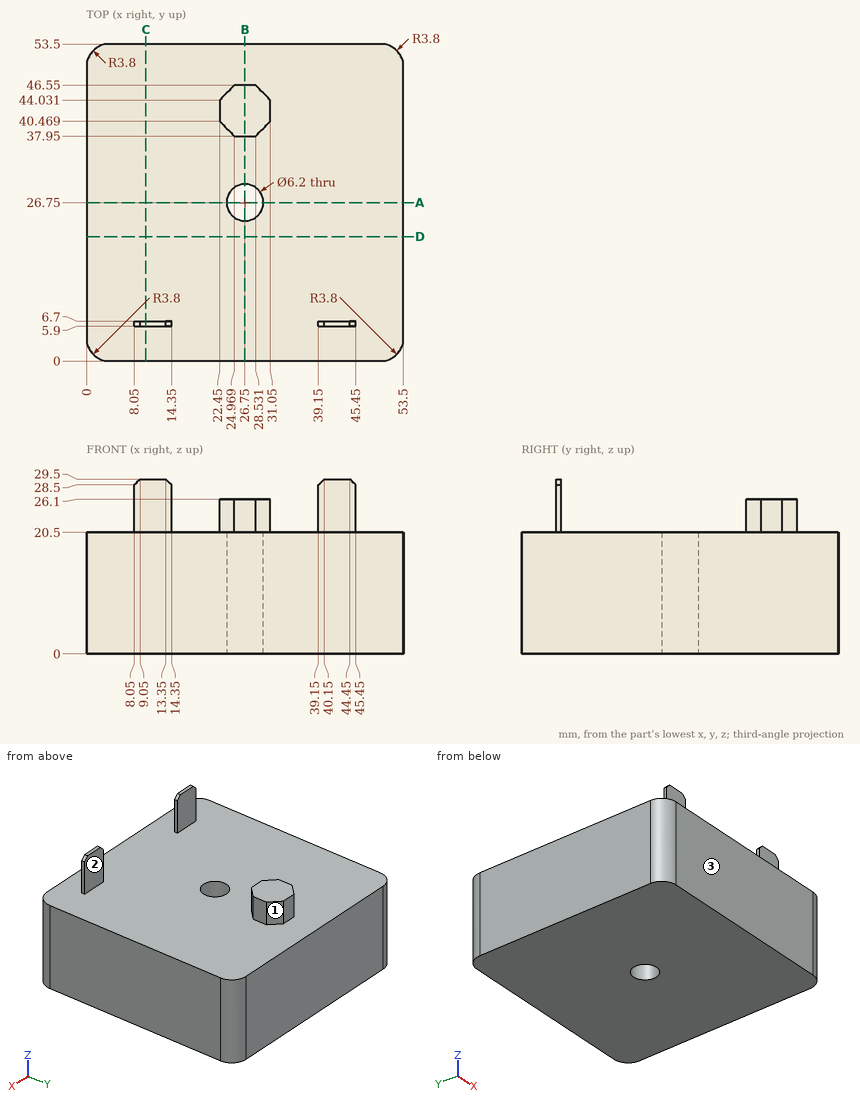
Answer from the drawing. Dimensions are ordinates in mm from the lowest x, y and z of the part. A direction names the side the tool comes from. Round coordinates to 2 decimals unless told otherwise and drop trailing zeros. Write each loop counter-clockwise with the first axis right and the second up, starting at its lowest first coordinate (ties: lowest second). Pieces come first, ordered by that corner, then holes.
1. The part is cut by section D-D, the plane y = 21. Determine the outline of the cut face in (x, z).
2. The part is cut by section A-A, the plane y = 26.75. Determine the outline of the cut face in (x, z).
3. The part is cut by section C-C, the plane x = 10. Determine the outline of the cut face in (y, z).
4. Which of the six approach directions +Z, -Z, +X, -X, +Y, -Y give full straight-line access (tool end or side, diameter ignored) to the marked faces 1, 2 and 3?
5. Straight lines are drawn through the part: L1, parallel to Y at x = 26.75, z = 8.5; L2, parallel to X at y = 26.5, z = 8; L3, parallel to Z at x = 16.5, y = 14. For each, find the intervals that lie inside material, in ascending order.
6. The part is cut by section B-B, the plane x = 26.75. Determine the outline of the cut face in (y, z).
7. Given pin 1 Ø1.8 at (y, z) = (43, 22) entering from +X; pin 2 Ø3 at (y, z) = (42, 23.5) entering from -X; pin 3 Ø1.9 at (x, z) = (11.5, 27) entering from -Y, each flat-ended and moving along its own axis, determine where each tip first touches the part or whether it passes through.
Values:
1. outline: (0, 0) - (53.5, 0) - (53.5, 20.5) - (0, 20.5) - close
2. outline: (0, 0) - (23.65, 0) - (23.65, 20.5) - (0, 20.5) - close; (29.85, 0) - (53.5, 0) - (53.5, 20.5) - (29.85, 20.5) - close
3. outline: (0, 0) - (53.5, 0) - (53.5, 20.5) - (6.7, 20.5) - (6.7, 29.5) - (5.9, 29.5) - (5.9, 20.5) - (0, 20.5) - close
4. face 1: +Z, +X, +Y
4. face 2: +Z, +X, -X, +Y
4. face 3: +Z, -Z, +X, -X, -Y
5. L1: y = 0 to 23.65, 29.85 to 53.5
5. L2: x = 0 to 23.66, 29.84 to 53.5
5. L3: z = 0 to 20.5
6. outline: (0, 0) - (23.65, 0) - (23.65, 20.5) - (0, 20.5) - close; (29.85, 0) - (53.5, 0) - (53.5, 20.5) - (46.55, 20.5) - (46.55, 26.1) - (37.95, 26.1) - (37.95, 20.5) - (29.85, 20.5) - close
7. pin 1: stops at x = 31.05
7. pin 2: stops at x = 22.45
7. pin 3: stops at y = 5.9
